Autodesk Inventor part; units mm, degrees
ref_plane "YZ Plane" through (0, 0, 0) normal (1, 0, 0) x (0, 1, 0)
ref_plane "XZ Plane" through (0, 0, 0) normal (0, 1, 0) x (-1, 0, 0)
ref_plane "XY Plane" through (0, 0, 0) normal (0, 0, 1) x (1, 0, 0)
sketch "Sketch1" plane through (0, 0, 0) normal (0, 0, 1) x (1, 0, 0)
  circle A0 centre (0, 0) radius 19.25
  circle A1 centre (0, 12.5) radius 1.5
  circle A2 centre (-10.8253, -6.25) radius 1.5
  circle A3 centre (10.8253, -6.25) radius 1.5
  circle A4 centre (0, 0) radius 5
  dimension "d0" = 38.5
  dimension "d1" = 3
  dimension "d4" = 360
  dimension "d6" = 12.5
  dimension "d7" = 10
extrude "Extrusion1" add sketch "Sketch1" along normal blind 5
sketch "Sketch2" plane through (0, 0, 5) normal (0, 0, 1) x (1, 0, 0)
  circle A0 centre (0, 12.5) radius 1.5
  circle A1 centre (10.8253, -6.25) radius 1.5
  circle A2 centre (-10.8253, -6.25) radius 1.5
  circle A3 centre (0, 12.5) radius 3
  circle A4 centre (10.8253, -6.25) radius 1.5
  circle A5 centre (10.8253, -6.25) radius 3
  circle A6 centre (-10.8253, -6.25) radius 3
  point P0 (0, 0)
  dimension "d10" = 6
  dimension "d11" = 6
  dimension "d12" = 6
extrude "Extrusion2" cut sketch "Sketch2" against normal blind 3 contours A0 | A1 | A2 | A3 | A5 | A6
properties part number "SJ018" material "ABS Plastic"
Source: CAD feature listing. Evaluate the final solid. Frame: model axes, mm. A direction names the side the tool comes from. Give positions to 0.01 mm unless a question says otherwise; leave off trailing zeros. Loops run counter-clockwise (first coordinate to the right, second up) from the corner with the lowest first, then second, coordinate; pieces in that order, holes last. Notation, with made-up numbers: (53, -38) -> (67, -38) arc R28 ccw to (67, -1) -> close; hole circle Ø2 at (10, 72.25). An arc over 180 degrees is marked (long way). Use a Markdown table: item, result. Add a question column.
1) First-contact query: pin 1 (5 mm diameter, centred on x = 10.83, y = -6.25, fed in from +Z); pin 2 (2 mm diameter, centred on x = 1.5, z = 4.5, fed in from +Y); pin 3 (1 mm diameter, centred on y = 3, z = 2, fed in from +X). Flat tips, straight axial feed; report the tip coordinate or a pass-through.
2) Line query: line 1 along Y through (x, z) = (0, 3.3); line 2 along X through (y, z) = (-8.5, 2.1); line 3 along Y through (x, z) = (-2, 3.55). Output: solid intervals per line, ascending. Write a range as [from, to].
3) Reachability of faces 4 (the face through (-1.08, 4.88, 2.46)), 5 (the face through (1, 14, 2)) from +Z, -Z, +X, -X, +Y, -Y: full face, straight path, thin tool, end or side. Return the list, or none.
4) Section query B-B, the plane x = 0. Return the cut outline in (y, z), then the cut area to 4 significant figures.
5) Pull-direction query (Y, two-part tool) for faces 1 (the face through (-12, -5, 2)), 2 (the face through (-15.28, 11.71, 2.46)), 3 (the face through (4, -4, 0)); classes: +Y half, -Y half, draft (parallel to the pull), parting line (faces both ways), or undercut.
6) Section query C-C, the plane x = -11. Return the cut outline in (y, z).
7) Section query D-D, the plane z = 3.7. Return the cut outline in (x, y), then the cut area to 3 significant figures.
8) Section query A-A, the plane y = 0. Return the cut outline in (x, z).
Numbers:
| question | item | result |
|---|---|---|
| 1 | pin 1 | stops at z = 2 |
| 1 | pin 2 | stops at y = 19.24 |
| 1 | pin 3 | stops at x = 19.09 |
| 2 | line 1 | y = [-19.25, -5], [5, 9.5], [15.5, 19.25] |
| 2 | line 2 | x = [-17.27, -12.81], [-8.84, 8.84], [12.81, 17.27] |
| 2 | line 3 | y = [-19.15, -4.58], [4.58, 10.26], [14.74, 19.15] |
| 3 | face 4 | +Z, -Z |
| 3 | face 5 | +Z |
| 4 | outline | (-19.25, 0) -> (-5, 0) -> (-5, 5) -> (-19.25, 5) -> close; (5, 0) -> (11, 0) -> (11, 2) -> (9.5, 2) -> (9.5, 5) -> (5, 5) -> close; (14, 0) -> (19.25, 0) -> (19.25, 5) -> (15.5, 5) -> (15.5, 2) -> (14, 2) -> close |
| 4 | area | 118.5 mm2 |
| 5 | face 1 | undercut |
| 5 | face 2 | parting line |
| 5 | face 3 | draft |
| 6 | outline | (-15.8, 0) -> (-7.74, 0) -> (-7.74, 2) -> (-9.24, 2) -> (-9.24, 5) -> (-15.8, 5) -> close; (-4.76, 0) -> (15.8, 0) -> (15.8, 5) -> (-3.26, 5) -> (-3.26, 2) -> (-4.76, 2) -> close |
| 7 | outline | circle Ø38.5 at (0, 0); hole circle Ø6 at (-10.83, -6.25); hole circle Ø10 at (0, 0); hole circle Ø6 at (0, 12.5); hole circle Ø6 at (10.83, -6.25) |
| 7 | area | 1,000 mm2 |
| 8 | outline | (-19.25, 0) -> (-5, 0) -> (-5, 5) -> (-19.25, 5) -> close; (5, 0) -> (19.25, 0) -> (19.25, 5) -> (5, 5) -> close |
